```python
from build123d import *

# Parameters (mm, degrees)
F1_DEPTH  = 45.72
F3_DEPTH  = 40.64
F5_DEPTH  = 25.4
F6_DEPTH  = 25.4
F7_DEPTH  = 25.4
F8_DEPTH  = 25.4
F9_DEPTH  = 2.54
F10_DEPTH = 2.54
F11_W     = 35.5600006878
F11_H     = 13.2107668169
F12_DEPTH = 2.54
F13_W     = 37.026392296
F13_H     = 12.4482874382
F14_DEPTH = 2.54
F17_DEPTH = 2.54
F18_DEPTH = 2.54
F19_W     = 34.2769082636
F19_H     = 15.8553607762
F20_DEPTH = 25.4


with BuildPart() as f1:
    # F0 (on Right) → F1 (new body)
    with BuildSketch(Plane.YZ):
        Polygon((-28.6284703761, 3.1933195423), (21.7250119895, 4.1742315516), (13.6597361416, 13.656382449), (-20.5631945282, 13.656382449), align=None)
        with BuildLine():
            Line((53.3399991691, -19.5213407278), (53.3399991691, 19.5213407278))
            Line((53.3399991691, 19.5213407278), (43.0870950222, 4.1742315516))
            Line((43.0870950222, 4.1742315516), (21.7250119895, 4.1742315516))
            Line((21.7250119895, 4.1742315516), (-28.6284703761, 3.1933195423))
            Line((-28.6284703761, 3.1933195423), (-62.7424120903, 3.1933195423))
            Line((-62.7424120903, 3.1933195423), (-73.3144581318, 0))
            Line((-73.3144581318, 0), (-50.7534816861, -19.5213407278))
            Line((-50.7534816861, -19.5213407278), (-36.8430949748, -19.5213407278))
            ThreePointArc((-36.8430949748, -19.5213407278), (-28.3196913078, -9.6037565649), (-19.7962876409, -19.5213407278))
            Line((-19.7962876409, -19.5213407278), (20.896082744, -19.5213407278))
            ThreePointArc((20.896082744, -19.5213407278), (28.6862896755, -10.0693031936), (36.4764966071, -19.5213407278))
            Line((36.4764966071, -19.5213407278), (53.3399991691, -19.5213407278))
        make_face()
    extrude(amount=F1_DEPTH)

    # F2 (on Right) → F3 (join)
    with BuildSketch(Plane.YZ):
        with BuildLine():
            ThreePointArc((20.7127835602, -19.8879390955), (28.5946400836, -26.5695137941), (36.4764966071, -19.8879390955))
            ThreePointArc((36.4764966071, -19.8879390955), (28.5946400836, -10.2776465209), (20.7127835602, -19.8879390955))
        make_face()
        with BuildLine():
            ThreePointArc((-36.8430912495, -19.704638049), (-28.1442910168, -27.4854506573), (-19.6129884571, -19.5213407278))
            ThreePointArc((-19.6129884571, -19.5213407278), (-28.3323258535, -9.8100174081), (-36.8430912495, -19.704638049))
        make_face()
    extrude(amount=F3_DEPTH)

    # F4: F1 across plane


with BuildPart() as f1_1:
    add(f1.part)
    add(f1.part.mirror(Plane.YZ))

    # F5 (cut): faces of the model
    f5_faces = [f1_1.faces().sort_by_distance(p)[0] for p in [
        (45.72, -3.0719009066, -4.1533515012),
        (40.64, -28.256328602, -18.6447266271),
    ]]
    extrude(f5_faces, amount=-F5_DEPTH, mode=Mode.SUBTRACT)

    # F6 (cut): a face of the model
    f6_faces = [f1_1.faces().sort_by_distance(p)[0] for p in [
        (40.64, 28.6216517019, -18.4204608425),
    ]]
    extrude(f6_faces, amount=-F6_DEPTH, mode=Mode.SUBTRACT)

    # F7 (cut): a face of the model
    f7_faces = [f1_1.faces().sort_by_distance(p)[0] for p in [
        (-45.72, -3.0719009066, -4.1533515012),
    ]]
    extrude(f7_faces, amount=-F7_DEPTH, mode=Mode.SUBTRACT)

    # F8 (cut): faces of the model
    f8_faces = [f1_1.faces().sort_by_distance(p)[0] for p in [
        (-40.64, 28.6216517019, -18.4204608425),
        (-40.64, -28.256328602, -18.6447266271),
    ]]
    extrude(f8_faces, amount=-F8_DEPTH, mode=Mode.SUBTRACT)

    # F9 (add): faces of the model
    f9_faces = [f1_1.faces().sort_by_distance(p)[0] for p in [
        (15.24, -28.256328602, -18.6447266271),
        (15.24, 28.6216517019, -18.4204608425),
    ]]
    extrude(f9_faces, amount=F9_DEPTH)

    # F10 (add): faces of the model
    f10_faces = [f1_1.faces().sort_by_distance(p)[0] for p in [
        (-15.24, 28.6216517019, -18.4204608425),
        (-15.24, -28.256328602, -18.6447266271),
    ]]
    extrude(f10_faces, amount=F10_DEPTH)

    # F11 (on face) → F12 (cut)
    with BuildSketch(Plane(origin=(0, -19.5021350286, 15.0328923789), x_dir=(1, 0, 0), z_dir=(0, -0.7920102634, 0.6105077744))):
        with Locations((-0.3665983677, -8.3433784743)):
            Rectangle(F11_W, F11_H)
    extrude(amount=-F12_DEPTH, mode=Mode.SUBTRACT)

    # F13 (on face) → F14 (cut)
    with BuildSketch(Plane(origin=(0, 14.6654159011, 12.4740289357), x_dir=(-1, 0, 0), z_dir=(0, 0.761723325, 0.6479024434))):
        with Locations((9.313e-07, -4.6719350962)):
            Rectangle(F13_W, F13_H)
    extrude(amount=-F14_DEPTH, mode=Mode.SUBTRACT)

    # F16 (on face) → F17 (cut)
    with BuildSketch(Plane(origin=(-20.32, 0, 0), x_dir=(0, -1, 0), z_dir=(-1, 0, 0))):
        Polygon((-13.6597361416, 13.656382449), (-21.7250119895, 4.1742315516), (28.6284703761, 3.1933195423), (20.5631945282, 13.656382449), align=None)
    extrude(amount=-F17_DEPTH, mode=Mode.SUBTRACT)

    # F15 (on face) → F18 (cut)
    with BuildSketch(Plane.YZ.offset(20.32)):
        Polygon((-20.5631945282, 13.656382449), (-28.6284703761, 3.1933195423), (21.7250119895, 4.1742315516), (13.6597361416, 13.656382449), align=None)
    extrude(amount=-F18_DEPTH, mode=Mode.SUBTRACT)

    # F19 (on face) → F20 (cut)
    with BuildSketch(Plane(origin=(0, 53.3399991691, 0), x_dir=(-1, 0, 0), z_dir=(0, 1, 0))):
        with Locations((-0.4582470283, 7.9276803881)):
            Rectangle(F19_W, F19_H)
    extrude(amount=-F20_DEPTH, mode=Mode.SUBTRACT)


solid = f1_1.part
```
The model under review builds one solid part; all positions refer to its coordinate system, in mm. A direction names the side the tool comes from. Round coordinates to 2 decimals unless told otherwise and drop trailing zeros. Write each loop counter-clockwise with the first axis right and the second up, starting at its lowest first coordinate (ties: lowest second). Pieces come first, ordered by that corner, then holes. Notation, with made-up numbers: (61.5, 70) -> (92.5, 70) arc R19 ccw to (92.5, 98) -> close; hole circle Ø2 at (42, 6.5). An arc over 180 degrees is marked (long way). Use CSV: the item, a comma, the result in double quotes.
Q1. Consider section A-A (z = 6). Give the boundary of the cut face in (x, y), then the cut area to 3 significant figures.
Checks:
outline,"(-20.32, 44.31) -> (-16.68, 44.31) -> (-16.68, 53.34) -> (-20.32, 53.34) -> close; (-17.78, -23.26) -> (17.41, -23.26) -> (17.41, -26.46) -> (17.78, -26.46) -> (17.78, 16.84) -> (-17.78, 16.84) -> close; (17.6, 44.31) -> (20.32, 44.31) -> (20.32, 53.34) -> (17.6, 53.34) -> close"
area,"1,480 mm²"
Q2. For faces 5 (the flat face through (0, 53.34, -5)), 6 (the flat face through (-16.68, 46, 4)), list the 3-axis set-ups (+Z, -Z, +X, -X, +Y, -Y) from which the entire face can be reached by the end or side of a thin tool; tool diameter is ignored.
Checks:
face 5,"+Z, -Z, +X, -X, +Y"
face 6,"+Y"
Q3. Consider section D-D (z = -12). Give the boundary of the cut face in (x, y), then the cut area to 3 significant figures.
Checks:
outline,"(-20.32, -59.45) -> (20.32, -59.45) -> (20.32, -34.28) -> (-20.32, -34.28) -> close; (-20.32, -22.36) -> (20.32, -22.36) -> (20.32, 23.5) -> (-20.32, 23.5) -> close; (-20.32, 33.87) -> (20.32, 33.87) -> (20.32, 53.34) -> (-20.32, 53.34) -> close; (-17.78, -34.01) -> (17.78, -34.01) -> (17.78, -22.47) -> (-17.78, -22.47) -> close; (-17.78, 23.62) -> (17.78, 23.62) -> (17.78, 33.57) -> (-17.78, 33.57) -> close"
area,"4,440 mm²"
Q4. Mouldability with a two-part tool opening along Y and no side actions: class faces 1 (the flat face through (0.284, -62.192, -9.624)), 2 (the cylindrical face through (0.25, 28.44, -26.57)), 3 (the cylindrical face through (0.25, 31.01, -10.65)), 4 (the flat face through (17.78, -5, 8)) as released by +Y, released by -Y, zero draft, split by the parting line, or undercut.
Checks:
face 1,"released by -Y"
face 2,"undercut"
face 3,"undercut"
face 4,"zero draft"
Q5. Consider section C-C (x = -9). State how many separate pieces and enclosed holes the cut face has, then the cut area to 3 significant figures.
Checks:
separate pieces,"2"
enclosed holes,"2"
area,"3,140 mm²"
Q6. To check wall thickness, follow probe 1 along X at (y, z) = (48, 4); probe 2 along Y at (x, z) = (-18, -17); probe 3 along Z at (x, y) = (7.5, 28.5). State the ranges of each line that lie inside material, in increasing order. Write a range as [from, to].
Checks:
probe 1,"[-20.32, -16.68], [17.6, 20.32]"
probe 2,"[-53.67, -36.85], [-19.79, 20.81], [36.56, 53.34]"
probe 3,"[-26.57, -10.28], [-10.07, 0]"
Q7. For pin 1 Ø4 at (y, z) = (8.5, 6) entering from +X; pin 2 Ø2 at (y, z) = (-9.5, -22) entering from +X; pin 3 Ø2 at (x, z) = (5, 0.5) entering from -Y; pin 4 Ø10.5 at (x, y) = (-6.5, -1.5) entering from +Z, all flat-tipped, find the tip position at first contact; note any pin that passes through.
Checks:
pin 1,"x = 17.78"
pin 2,"through"
pin 3,"y = -73.31"
pin 4,"z = 13.66"
Q8. Consider section B-B (y = -34.5). Give the boundary of the cut face in (x, z), then the cut area to 3 significant figures.
Checks:
outline,"(-20.32, -12.21) -> (20.32, -12.21) -> (20.32, 3.19) -> (-20.32, 3.19) -> close; (-17.78, -24.8) -> (17.78, -24.8) -> (17.78, -12.47) -> (-17.78, -12.47) -> close"
area,"1,060 mm²"
